```python
from build123d import *

# Parameters (mm, degrees)
SKETCH1_W           = 58.7
SKETCH1_H           = 14.5
BOSS_EXTRUDE1_DEPTH = 2
SKETCH2_W           = 1.907537222
SKETCH2_H           = 8.6
BOSS_EXTRUDE2_DEPTH = 4.3
SKETCH3_W           = 2.3
SKETCH3_H           = 8.6
BOSS_EXTRUDE3_DEPTH = 4.3
FILLET3_R           = 2
SKETCH4_W           = 0.949738238
SKETCH4_H           = 9
BOSS_EXTRUDE4_DEPTH = 12
SKETCH5_W           = 14
SKETCH5_H           = 9.016953004
BOSS_EXTRUDE5_DEPTH = 10
FILLET4_R           = 5.5
CUT_EXTRUDE1_DEPTH  = 12
SKETCH8_W           = 2.580145407
SKETCH8_H           = 9.016953004
SKETCH8_W_2         = 1.5
BOSS_EXTRUDE6_DEPTH = 2
SKETCH9_W           = 1.920869139
SKETCH9_H           = 1.685794619
SKETCH9_H_2         = 1.68579462
BOSS_EXTRUDE7_DEPTH = 3
FILLET6_R           = 3
FILLET9_R           = 3
FILLET11_R          = 1
FILLET12_R          = 1


with BuildPart() as part:
    # Sketch1 → Boss-Extrude1 (new body)
    with BuildSketch(Plane.XY):
        with Locations((15.900667763, -7.24741023)):
            Rectangle(SKETCH1_W, SKETCH1_H)
        with Locations((15.900667763, 7.25258977)):
            Rectangle(SKETCH1_W, SKETCH1_H)
    extrude(amount=BOSS_EXTRUDE1_DEPTH)

    # Sketch2 → Boss-Extrude2 (add)
    with BuildSketch(Plane.XY.offset(2)):
        with Locations((44.296899152, 0)):
            Rectangle(SKETCH2_W, SKETCH2_H)
    extrude(amount=-BOSS_EXTRUDE2_DEPTH)

    # Sketch3 → Boss-Extrude3 (add)
    with BuildSketch(Plane(origin=(45.250667763, 0, 0), x_dir=(0, 0, -1), z_dir=(1, 0, 0))):
        with Locations((1.15, 0)):
            Rectangle(SKETCH3_W, SKETCH3_H)
    extrude(amount=BOSS_EXTRUDE3_DEPTH)

    # Fillet3
    fillet3_edges = [part.edges().sort_by_distance(p)[0] for p in [
        (43.343130541, 0, -2.3),
    ]]
    fillet(fillet3_edges, radius=FILLET3_R)

    # Sketch4 → Boss-Extrude4 (add)
    with BuildSketch(Plane(origin=(0, 0, 0), x_dir=(-1, 0, 0), z_dir=(0, 0, -1))):
        with Locations((12.974463118, 0.00258977)):
            Rectangle(SKETCH4_W, SKETCH4_H)
    extrude(amount=BOSS_EXTRUDE4_DEPTH)

    # Sketch5 → Boss-Extrude5 (add)
    with BuildSketch(Plane.ZY.offset(13.449332237)):
        with Locations((-5, -0.005886732)):
            Rectangle(SKETCH5_W, SKETCH5_H)
    extrude(amount=BOSS_EXTRUDE5_DEPTH)

    # Fillet4
    # the kernel refuses this fillet: 5.5 mm, written as the material it takes off along each edge
    with BuildSketch(Plane(origin=(-23.449332237, -18.264363234, -12), x_dir=(1, 0, 0), z_dir=(0, 1, 0))) as fillet4_piece_1:
        with BuildLine():
            CenterArc((FILLET4_R, -FILLET4_R), FILLET4_R, 90, 90)
            Line((0, -FILLET4_R), (0, 0))
            Line((0, 0), (FILLET4_R, 0))
        make_face()
    extrude(amount=36.516953004, mode=Mode.SUBTRACT)
    with BuildSketch(Plane(origin=(-12.499593999, -18.24741023, -12), x_dir=(-1, 0, 0), z_dir=(0, 1, 0))) as fillet4_piece_2:
        with BuildLine():
            CenterArc((FILLET4_R, FILLET4_R), FILLET4_R, 180, 90)
            Line((0, FILLET4_R), (0, 0))
            Line((0, 0), (FILLET4_R, 0))
        make_face()
    extrude(amount=36.5, mode=Mode.SUBTRACT)

    # Sketch7 → Cut-Extrude1 (cut)
    with BuildSketch(Plane(origin=(0, 4.50258977, 0), x_dir=(1, 0, 0), z_dir=(0, 1, 0))):
        with BuildLine():
            ThreePointArc((-15.03934254, 6.5), (-17.974463118, 9.435120578), (-20.909583696, 6.5))
            Line((-20.909583696, 6.5), (-15.03934254, 6.5))
        make_face()
        with BuildLine():
            Line((-15.03934254, 6.5), (-20.909583696, 6.5))
            ThreePointArc((-20.909583696, 6.5), (-17.974463118, 3.564879422), (-15.03934254, 6.5))
        make_face()
        with BuildLine():
            ThreePointArc((-15.03934254, 6.5), (-17.974463118, 3.564879422), (-20.909583696, 6.5))
            Line((-20.909583696, 6.5), (-20.909583696, -2))
            Line((-20.909583696, -2), (-15.03934254, -2))
            Line((-15.03934254, -2), (-15.03934254, 6.5))
        make_face()
    extrude(amount=-CUT_EXTRUDE1_DEPTH, mode=Mode.SUBTRACT)

    # Sketch8 → Boss-Extrude6 (add)
    with BuildSketch(Plane.ZY.offset(23.449332237)):
        with Locations((-2.790072703, -0.005886732)):
            Rectangle(SKETCH8_W, SKETCH8_H)
        with Locations((1.25, -0.005886732)):
            Rectangle(SKETCH8_W_2, SKETCH8_H)
    extrude(amount=BOSS_EXTRUDE6_DEPTH)

    # Sketch9 → Boss-Extrude7 (add)
    with BuildSketch(Plane(origin=(0, 0, 0), x_dir=(-1, 0, 0), z_dir=(0, 0, -1))):
        with Locations((11.550124457, -3.589191377)):
            Rectangle(SKETCH9_W, SKETCH9_H)
        with Locations((11.539159429, 3.65969246)):
            Rectangle(SKETCH9_W, SKETCH9_H_2)
    extrude(amount=BOSS_EXTRUDE7_DEPTH)

    # Fillet6
    # the kernel refuses this fillet: 3 mm, written as the material it takes off along each edge
    with BuildSketch(Plane(origin=(-10.589689887, 4.241056538, -3), x_dir=(-1, 0, 0), z_dir=(0, -1, 0))) as fillet6_piece_1_section:
        with BuildLine():
            CenterArc((3, -2.794940242), FILLET6_R, 111.307014795, 68.692985205)
            Line((0, -2.794940242), (0, 0))
            Line((0, 0), (1.909904112, 0))
        make_face()
    fillet6_piece_1 = extrude(amount=15.660495829, mode=Mode.PRIVATE)
    fillet6_piece_1 = split(fillet6_piece_1, bisect_by=Plane(origin=(-11.107813793, 2.81679515, -1.901033535), z_dir=(0, -1, 0)), keep=Keep.TOP, mode=Mode.PRIVATE)
    add(fillet6_piece_1, mode=Mode.SUBTRACT)
    with BuildSketch(Plane(origin=(-10.57872486, 11.500570097, -3), x_dir=(-1, 0, 0), z_dir=(0, -1, 0))) as fillet6_piece_2:
        with BuildLine():
            CenterArc((3, -2.799192131), FILLET6_R, 111.082404826, 68.917595174)
            Line((0, -2.799192131), (0, 0))
            Line((0, 0), (1.920869139, 0))
        make_face()
    extrude(amount=15.681755273, mode=Mode.SUBTRACT)

    # Fillet9
    # the kernel refuses this fillet: 3 mm, written as the material it takes off along each edge
    with BuildSketch(Plane(origin=(49.550667763, 11.592976073, -2.3), x_dir=(-1, 0, 0), z_dir=(0, -1, 0))) as fillet9_piece_1:
        with BuildLine():
            CenterArc((2.917190429, -3), FILLET9_R, 90, 76.506601178)
            Line((0, -2.3), (-0.058343809, -2.286))
            ThreePointArc((-0.058343809, -2.286), (-0.06, -1.15), (-0.06, 0))
            Line((-0.06, 0), (0, 0.06))
            Line((0, 0.06), (2.917190429, 0.06))
            Line((2.917190429, 0.06), (2.917190429, 0))
        make_face()
    extrude(amount=23.185952146, mode=Mode.SUBTRACT)

    # Fillet11
    fillet11_edges = [part.edges().sort_by_distance(p)[0] for p in [
        (-25.449332237, -0.005886732, -4.080145407),
        (-25.449332237, -4.514363234, -2.790072704),
        (-25.449332237, -0.005886732, -1.5),
        (-25.449332237, 4.50258977, -2.790072704),
    ]]
    fillet(fillet11_edges, radius=FILLET11_R)

    # Fillet12
    fillet12_edges = [part.edges().sort_by_distance(p)[0] for p in [
        (-25.449332237, 4.50258977, 1.25),
        (-25.449332237, -0.005886732, 0.5),
        (-25.449332237, -4.514363234, 1.25),
    ]]
    fillet(fillet12_edges, radius=FILLET12_R)


solid = part.part
```
The model under review builds one solid part; all positions refer to its coordinate system, in mm. A direction names the side the tool comes from. Round coordinates to 2 decimals unless told otherwise and drop trailing zeros. Loops run counter-clockwise (first coordinate to the right, second up) from the corner with the lowest first, then second, coordinate; pieces in that order, holes last. Notation, with made-up numbers: M 27,74.25 L 79,74.25 A33 cw 79,109.25 Z; hole C 78,16.5 d10. An arc over 180 degrees is marked long. Put each result on its own line as item: value.
Q1. For pin 1 (1.2 mm diameter, centred on y = -1.5, z = -5.5, fed in from -X); pin 2 (1 mm diameter, centred on x = -13, z = -6.5, fed in from -Y); pin 3 (0.6 mm diameter, centred on x = -11.5, z = -1.5, fed in from -Y), all flat-tipped, find the tip position at first contact; note any pin that passes through.
Result set:
pin 1: stops at x = -23.45
pin 2: stops at y = -4.51
pin 3: stops at y = -4.43
Q2. Consider section A-A, the plane x = 6.5. Give the boundary of the cut face in (y, z), then the cut area to 3 significant figures.
Result set:
outline: M -14.5,0 L 14.5,0 L 14.5,2 L -14.5,2 Z
area: 58.0 mm²
Q3. Mouldability with a two-part tool opening along Z and no side actions: class faces 6 (the flat face through (-23.449, 0, -1)), 7 (the flat face through (-12, -4.432, -1)), 8 (the flat face through (-23, 0, 2)), 9 (the cylindrical face through (43.945, 0.06, -1.73)) as released by +Z, released by -Z, zero draft, split by the parting line, or undercut.
Result set:
face 6: undercut
face 7: zero draft
face 8: released by +Z
face 9: released by -Z
Q4. Machinability: for faces 1 (the flat face through (-15.039, 0, -2)), 2 (the flat face through (47, 0, 0)), 3 (the flat face through (46, 4.3, -1)), 4 (the flat face through (-12, 2.817, -1)), 5 (the flat face through (46, -4.3, -1)), which of the approach directions +Z, -Z, +X, -X, +Y, -Y give a long, thin tool a straight path to every point of the face, cutting with its end or side? Answer none if there is none.
Result set:
face 1: +Z, +Y, -Y
face 2: +Z, +X, +Y, -Y
face 3: -Z, +X, +Y
face 4: -Z
face 5: -Z, +X, -Y
Q5. To check wall thickness, follow L1, parallel to X at y = 0.75, z = -1; L2, parallel to Z at x = 9, y = -4; L3, parallel to X at y = -3.25, z = -7.75. State the ranges of each line that lie inside material, in increasing order.
Result set:
L1: x = -23.45 to -20.91, -15.04 to -12.5, 43.47 to 49.11
L2: z = 0 to 2
L3: x = -23.31 to -20.63, -15.32 to -12.64
